Autodesk Inventor part; units mm, degrees
ref_plane "YZ Plane" through (0, 0, 0) normal (1, 0, 0) x (0, 1, 0)
ref_plane "XZ Plane" through (0, 0, 0) normal (0, 1, 0) x (-1, 0, 0)
ref_plane "XY Plane" through (0, 0, 0) normal (0, 0, 1) x (1, 0, 0)
sketch "Sketch1" plane through (0, 0, 0) normal (0, 0, 1) x (1, 0, 0)
  line L0 (-32.5, -42.5) -> (32.5, -42.5)
  line L1 (32.5, -42.5) -> (32.5, 42.5)
  line L2 (32.5, 42.5) -> (-32.5, 42.5)
  line L3 (-32.5, 42.5) -> (-32.5, -42.5)
  line L4 (-32.5, -42.5) -> (32.5, 42.5) construction
  line L5 (32.5, -42.5) -> (-32.5, 42.5) construction
  line L6 (15.25, -15.25) -> (-15.25, -15.25)
  line L7 (-15.25, -15.25) -> (-15.25, 15.25)
  line L8 (-15.25, 15.25) -> (15.25, 15.25)
  line L9 (15.25, 15.25) -> (15.25, -15.25)
  line L10 (15.25, -15.25) -> (-15.25, 15.25) construction
  line L11 (-15.25, -15.25) -> (15.25, 15.25) construction
  point P0 (0, 0)
  dimension "d154" = 65
  dimension "d155" = 85
  dimension "d172" = 30.5
extrude "Plate5" add sketch "Sketch1" along normal blind 3
sketch "Sketch9" plane through (0, 0, 3) normal (0, 0, 1) x (1, 0, 0)
  circle A0 centre (25, -35) radius 4.5
  line L0 (25, 35) -> (-25, 35) construction
  line L1 (-25, 35) -> (-25, -35) construction
  line L2 (-25, -35) -> (25, -35) construction
  line L3 (25, -35) -> (25, 35) construction
  line L4 (25, 35) -> (-25, -35) construction
  line L5 (-25, 35) -> (25, -35) construction
  circle A1 centre (-25, -35) radius 4.5
  circle A2 centre (25, 35) radius 4.5
  circle A3 centre (-25, 35) radius 4.5
  point P0 (0, 0)
  dimension "d173" = 70
  dimension "d174" = 9
  dimension "d175" = 50
extrude "Cut2" cut sketch "Sketch9" against normal blind 3
fillet "Corner Round1" radius 6 4 edges at (32.5, 42.5, 1.5) (-32.5, 42.5, 1.5) (-32.5, -42.5, 1.5) (32.5, -42.5, 1.5)
properties part number "PNS 760 FDS 1200 FLANGE 3" material "Stainless Steel"
CAD build for the part. Positions are in the model's coordinates, mm. A direction names the side the tool comes from. Round coordinates to 2 decimals unless told otherwise and drop trailing zeros. Order: outer loops, then holes, each group sorted by start corner. A loop starts at its lowest first (then second) coordinate and runs counter-clockwise, first axis right, second up. Notation, with made-up numbers: M 20.5,43 L 32.5,43 A11 cw 32.5,55 Z; hole C -26.75,57 d10. An arc over 180 degrees is marked long. Use one line per item in the form item = value.
Q1. Flat gauge pin, fed straight in: P1, Ø7, axis at x = 25, y = 35, coming from the -Z side. Where does the tip first touch, or does it go through?
Recorded:
P1 = through
Q2. Which spindle directions (+Z, -Z, +X, -X, +Y, -Y) get a long thin tool onto all of the face, cutting with end or side? Do faces 1 (the flat face through (0, -42.5, 1)), 2 (the flat face through (-15.25, 0, 1)). Say none if no direction does.
Recorded:
face_1 = +Z, -Z, +X, -X, -Y
face_2 = +Z, -Z
Q3. Saw through at D-D on y = -35. Give the cut face in (x, z), then the cut area to 3 significant figures.
Recorded:
outline = M -32.5,0 L -29.5,0 L -29.5,3 L -32.5,3 Z; M -20.5,0 L 20.5,0 L 20.5,3 L -20.5,3 Z; M 29.5,0 L 32.5,0 L 32.5,3 L 29.5,3 Z
area = 141 mm^2
Q4. Saw through at A-A on y = 0.5. Give the cut face in (x, z), then the cut area to 4 significant figures.
Recorded:
outline = M -32.5,0 L -15.25,0 L -15.25,3 L -32.5,3 Z; M 15.25,0 L 32.5,0 L 32.5,3 L 15.25,3 Z
area = 103.5 mm^2
Q5. Saw through at B-B on x = 25. Give the cut face in (y, z).
Recorded:
outline = M -42.5,0 L -39.5,0 L -39.5,3 L -42.5,3 Z; M -30.5,0 L 30.5,0 L 30.5,3 L -30.5,3 Z; M 39.5,0 L 42.5,0 L 42.5,3 L 39.5,3 Z
Q6. Two-plate mould, pull along X, no slides. Class faces 3 (the flat face through (0, 19, 0)), 4 (the cylindrical face through (-25.98, 30.61, 1.52)), 5 (the cylindrical face through (-30.696, 40.789, 1.521)), 6 (the cylindrical face through (30.789, 40.696, 1.521)): +X half, -X half, draft (parallel to the pull), parting line (faces both ways), or undercut.
Recorded:
face_3 = draft
face_4 = undercut
face_5 = -X half
face_6 = +X half
Q7. Probe L1, parallel to Y at x = -25, z = 1; L2, parallel to Y at x = -12.5, z = 2.4; L3, parallel to Y at x = 28, z = 0.3. List the from-to ranges inside material, lowest first.
Recorded:
L1 = -42.5 to -39.5, -30.5 to 30.5, 39.5 to 42.5
L2 = -42.5 to -15.25, 15.25 to 42.5
L3 = -42.31 to -38.35, -31.65 to 31.65, 38.35 to 42.31
Q8. Saw through at C-C on z = 1. Give the cut face in (x, y).
Recorded:
outline = M -32.5,-36.5 A6 ccw -26.5,-42.5 L 26.5,-42.5 A6 ccw 32.5,-36.5 L 32.5,36.5 A6 ccw 26.5,42.5 L -26.5,42.5 A6 ccw -32.5,36.5 Z; hole C -25,-35 d9; hole C -25,35 d9; hole M -15.25,-15.25 L 15.25,-15.25 L 15.25,15.25 L -15.25,15.25 Z; hole C 25,-35 d9; hole C 25,35 d9
